from build123d import *

# Parameters (mm, degrees)
F1_DEPTH = 7
F2_W     = 6
F2_H     = 4.91947
F3_DEPTH = 3.288103
F5_DEPTH = 7.001


with BuildPart() as f1:
    # F0 (on Right) → F1 (new body)
    with BuildSketch(Plane.YZ):
        with BuildLine():
            Line((-3.353103, 0.58162), (-0.066, 0.58162))
            Line((-0.066, 0.58162), (-0.066, 12.58162))
            ThreePointArc((-0.066, 12.58162), (-0.773107, 12.288727), (-1.066, 11.58162))
            Line((-1.066, 11.58162), (-1.066, 9.336664))
            ThreePointArc((-1.066, 9.336664), (-1.131912, 8.979622), (-1.32096, 8.669645))
            ThreePointArc((-1.32096, 8.669645), (-2.578651, 6.838208), (-3.329772, 4.74733))
            ThreePointArc((-3.329772, 4.74733), (-3.347253, 4.640585), (-3.353103, 4.532576))
            Line((-3.353103, 4.532576), (-3.353103, 0.58162))
        make_face()
    extrude(amount=F1_DEPTH)

    # F2 (on face) → F3 (cut, through all)
    with BuildSketch(Plane(origin=(0, -0.066, 0), x_dir=(-1, 0, 0), z_dir=(0, 1, 0))):
        with Locations((-3.5, 9.371885)):
            Rectangle(F2_W, F2_H)
    extrude(amount=-F3_DEPTH, mode=Mode.SUBTRACT)

    # F4 (on face) → F5 (cut, through all)
    with BuildSketch(Plane.YZ.offset(7)):
        with BuildLine():
            Line((-1.709552, 4.885615), (-1.709552, 0.58162))
            Line((-1.709552, 0.58162), (-0.066, 0.58162))
            Line((-0.066, 0.58162), (-0.066, 2.014811))
            Line((-0.066, 2.014811), (-0.066, 7.394113))
            ThreePointArc((-0.066, 7.394113), (-1.262072, 6.3851), (-1.709552, 4.885615))
        make_face()
    extrude(amount=-F5_DEPTH, mode=Mode.SUBTRACT)


solid = f1.part
The listing builds one solid part. Answer for the finished solid, in the listing's coordinates (mm). A direction names the side the tool comes from. Give positions to 0.01 mm unless a question says otherwise; leave off trailing zeros. Order: outer loops, then holes, each group sorted by start corner. A loop starts at its lowest first (then second) coordinate and runs counter-clockwise, first axis right, second up. Notation, with made-up numbers: (55.25, 22.5) - (62.25, 22.5) arc R22 ccw to (62.25, 32.5) - close; hole circle Ø6 at (86, 5). An arc over 180 degrees is marked (long way). Answer as CSV lines item,"result".
Q1. A cutting plane is placed at C-C, the plane y = -1.55. Determine the outline of the cut face in (x, z), and give its area (3 significant figures).
Answer key:
outline,"(0, 5.81) - (7, 5.81) - (7, 8.4) - (6.5, 8.4) - (6.5, 6.91) - (0.5, 6.91) - (0.5, 8.4) - (0, 8.4) - close"
area,"9.23 mm^2"
Q2. Determine the mould class of faces 1 (the face through (3.451, -0.765, 12.296)), 2 (the face through (3, -3.353, 3)), 3 (the face through (3.5, -0.5, 11.832)) for opening direction Z: pulls with the +Z half, pulls with the -Z half, needs draft (parallel to the pull), parting line crosses it, or undercut.
Answer key:
face 1,"pulls with the +Z half"
face 2,"needs draft"
face 3,"undercut"
Q3. Which of the six approach directions +Z, -Z, +X, -X, +Y, -Y give full straight-line access (tool end or side, diameter ignored) to faces 4 (the face through (3.45, -2.78, 6.42)), 5 (the face through (6.5, -0.7, 8.8)), 6 (the face through (4, -1.71, 3))?
Answer key:
face 4,"+Z, +X, -X, -Y"
face 5,"+Y, -Y"
face 6,"-Z, +X, -X, +Y"
Q4. Straight lines are drawn through the part: L1, parallel to Y at x = 2.75, z = 1; L2, parallel to Z at x = 3, y = -0.15; L3, parallel to Z at x = 2, y = -2.05. For each, find the intervals that lie inside material, in ascending order.
Answer key:
L1,"y = -3.35 to -1.71"
L2,"z = 11.83 to 12.58"
L3,"z = 0.58 to 6.91"
Q5. A cutting plane is placed at A-A, the plane z = 10.5. Determine the outline of the cut face in (x, y).
Answer key:
outline,"(0, -1.07) - (0.5, -1.07) - (0.5, -0.07) - (0, -0.07) - close; (6.5, -1.07) - (7, -1.07) - (7, -0.07) - (6.5, -0.07) - close"
Q6. A cutting plane is placed at D-D, the plane z = 8. Determine the outline of the cut face in (x, y).
Answer key:
outline,"(0, -1.86) - (0.5, -1.86) - (0.5, -0.07) - (0, -0.07) - close; (6.5, -1.86) - (7, -1.86) - (7, -0.07) - (6.5, -0.07) - close"
Q7. Each of these flat-tipped pins is pushed along its axis until it touches: pin 1 Ø1.3 at (x, z) = (2.5, 2) entering from +Y; pin 2 Ø1.5 at (x, y) = (2, -1.5) entering from +Z; pin 3 Ø3 at (x, z) = (4.5, 7) entering from -Y. Where does it stop, or does it pass through?
Answer key:
pin 1,"stops at y = -1.71"
pin 2,"stops at z = 12.31"
pin 3,"stops at y = -3.13"
Q8. A cutting plane is placed at B-B, the plane x = 5.5. Determine the outline of the cut face in (y, z).
Answer key:
outline,"(-3.35, 0.58) - (-1.71, 0.58) - (-1.71, 4.89) arc R2.74 cw to (-0.81, 6.91) - (-2.54, 6.91) arc R8.67 ccw to (-3.33, 4.75) arc R1 ccw to (-3.35, 4.53) - close; (-1.03, 11.83) - (-0.07, 11.83) - (-0.07, 12.58) arc R1 ccw to start"
